Verification items for the finished model (mm, model axes). Face numbers are marked on the shaded views. A direction names the side the tool comes from. Give positions to 0.01 mm unless a question says otherwise; leave off trailing zeros. Loops run counter-clockwise (first coordinate to the right, second up) from the corner with the lowest first, then second, coordinate; pieces in that order, holes last. Notation, with made-up numbers: (4, 78.5) -> (29, 78.5) arc R22 cw to (29, 89.5) -> close; hole circle Ø8 at (46.5, 21.25). An arc over 180 degrees is marked (long way). Answer in a Markdown table with one row per item. Add a question column.
Q1. Section check D-D on y = -20. Enter the section's corners in (x, z), and give its area (3 significant figures).
Q2. Section check A-A on x = 0. Enter the section's corners in (y, z).
Q3. Gauge pin test, flat ends, axial feed: P1, Ø1, axis at x = -12.5, z = -17, coming from the +Y side; P2, Ø6, axis at y = -17.5, z = -27, coming from the +X side; P3, Ø8, axis at y = 9.5, z = -24.5, coming from the -X side; P4, Ø18, axis at x = 0, y = 0, coming from the -Z side. Record the tip position at first contact, or that the pin passes through.
Q4. Set-up check for the marked faces 4, 5 and 6: record each of +Z, -Z, +X, -X, +Y, -Y from which the full face is reachable in a straight line by a thin tool's end or side.
Q5. Release check for a two-part mould opening along X. For the marked faces 1, 2 and 3 record: pulls with the +X half, pulls with the -X half, needs draft (parallel to the pull), parting line crosses it, or undercut.
Q6. Section check C-C on z = -1.75. Enter the section's corners in (x, y) (3 decimals).
Q7. Material ranges on probe 1 along Y at (x, z) = (24, -8.25); probe 2 along X at (y, z) = (3, -5.25); probe 3 along X at (y, z) = (10.5, -26), recorded low to high.
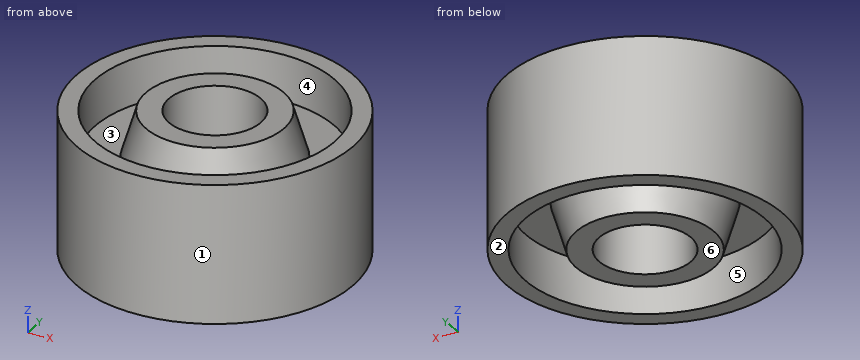
```python
from build123d import *

# Parameters (mm, degrees)
IZIM1_R                     = 30
Y_KSEKLIK_EKSTR_ZYON1_DEPTH = 30
IZIM2_R                     = 26
KES_EKSTR_ZYON1_DEPTH       = 10
IZIM3_R                     = 26
KES_EKSTR_ZYON2_DEPTH       = 10
IZIM4_R                     = 10
KES_EKSTR_ZYON3_DEPTH       = 10
IZIM6_R                     = 15
Y_KSEKLIK_EKSTR_ZYON3_DEPTH = 10
IZIM7_R                     = 10
KES_EKSTR_ZYON4_DEPTH       = 10
IZIM8_R                     = 15
Y_KSEKLIK_EKSTR_ZYON4_DEPTH = 10
IZIM9_R                     = 10
KES_EKSTR_ZYON5_DEPTH       = 10


with BuildPart() as part:
    # Çizim1 → Yükseklik-Ekstrüzyon1 (new body)
    with BuildSketch(Plane.XY):
        Circle(IZIM1_R)
    extrude(amount=-Y_KSEKLIK_EKSTR_ZYON1_DEPTH)

    # Çizim2 → Kes-Ekstrüzyon1 (cut)
    with BuildSketch(Plane.XY):
        Circle(IZIM2_R)
    extrude(amount=-KES_EKSTR_ZYON1_DEPTH, mode=Mode.SUBTRACT)

    # Çizim3 → Kes-Ekstrüzyon2 (cut)
    with BuildSketch(Plane(origin=(0, 0, -30), x_dir=(-1, 0, 0), z_dir=(0, 0, -1))):
        Circle(IZIM3_R)
    extrude(amount=-KES_EKSTR_ZYON2_DEPTH, mode=Mode.SUBTRACT)

    # Çizim4 → Kes-Ekstrüzyon3 (cut)
    with BuildSketch(Plane.XY.offset(-10)):
        Circle(IZIM4_R)
    extrude(amount=-KES_EKSTR_ZYON3_DEPTH, mode=Mode.SUBTRACT)

    # Çizim6 → Yükseklik-Ekstrüzyon3 (add)
    with BuildSketch(Plane.XY.offset(-10)):
        Circle(IZIM6_R)
    extrude(amount=Y_KSEKLIK_EKSTR_ZYON3_DEPTH)

    # Çizim7 → Kes-Ekstrüzyon4 (cut)
    with BuildSketch(Plane.XY):
        Circle(IZIM7_R)
    extrude(amount=-KES_EKSTR_ZYON4_DEPTH, mode=Mode.SUBTRACT)

    # Çizim8 → Yükseklik-Ekstrüzyon4 (add)
    with BuildSketch(Plane(origin=(0, 0, -20), x_dir=(-1, 0, 0), z_dir=(0, 0, -1))):
        Circle(IZIM8_R)
    extrude(amount=Y_KSEKLIK_EKSTR_ZYON4_DEPTH)

    # Çizim9 → Kes-Ekstrüzyon5 (cut)
    with BuildSketch(Plane(origin=(0, 0, -30), x_dir=(-1, 0, 0), z_dir=(0, 0, -1))):
        Circle(IZIM9_R)
    extrude(amount=-KES_EKSTR_ZYON5_DEPTH, mode=Mode.SUBTRACT)

    # Çizim12 → Döndür1 (revolve)
    with BuildSketch(Plane(origin=(0, 0, 0), x_dir=(0, 0, -1), z_dir=(1, 0, 0))):
        Polygon((10, 18), (0, 15), (10, 15), align=None)
    d_nd_r1 = revolve(axis=Axis((0, 0, 0), (0, 0, -1)))

    # Aynalama1: Döndür1 across plane
    add(d_nd_r1.mirror(Plane.XY.offset(-15)))


solid = part.part
```
Taken from the geometry:
| question | item | result |
|---|---|---|
| 1 | outline | (-22.36, -30) -> (-16.61, -30) -> (-16.61, -20) -> (16.61, -20) -> (16.61, -30) -> (22.36, -30) -> (22.36, 0) -> (16.61, 0) -> (16.61, -10) -> (-16.61, -10) -> (-16.61, 0) -> (-22.36, 0) -> close |
| 1 | area | 677 mm² |
| 2 | outline | (-30, -30) -> (-26, -30) -> (-26, -20) -> (-18, -20) -> (-15, -30) -> (-10, -30) -> (-10, 0) -> (-15, 0) -> (-18, -10) -> (-26, -10) -> (-26, 0) -> (-30, 0) -> close; (10, -30) -> (15, -30) -> (18, -20) -> (26, -20) -> (26, -30) -> (30, -30) -> (30, 0) -> (26, 0) -> (26, -10) -> (18, -10) -> (15, 0) -> (10, 0) -> close |
| 3 | P1 | stops at y = 27.5 |
| 3 | P2 | stops at x = 26.26 |
| 3 | P3 | stops at x = -29.49 |
| 3 | P4 | passes through |
| 4 | face 4 | +Z |
| 4 | face 5 | -Z |
| 4 | face 6 | -Z, +X, -X, +Y, -Y |
| 5 | face 1 | parting line crosses it |
| 5 | face 2 | needs draft |
| 5 | face 3 | undercut |
| 6 | outline | circle Ø60 at (0, 0); circle Ø31.05 at (0, 0); hole circle Ø52 at (0, 0); hole circle Ø20 at (0, 0) |
| 7 | probe 1 | y = -18 to -10, 10 to 18 |
| 7 | probe 2 | x = -29.85 to -25.83, -16.3 to -9.54, 9.54 to 16.3, 25.83 to 29.85 |
| 7 | probe 3 | x = -28.1 to -23.79, -12.34 to 12.34, 23.79 to 28.1 |
